```python
from build123d import *

# Parameters (mm, degrees)
BOSS_EXTRUDE2_DEPTH = 5
SKETCH5_R           = 4
BOSS_EXTRUDE3_DEPTH = 7
SKETCH6_R           = 15.5
CUT_EXTRUDE1_DEPTH  = 4
SKETCH7_R           = 1.8
CUT_EXTRUDE2_DEPTH  = 4
CUT_EXTRUDE3_DEPTH  = 6
CUT_EXTRUDE4_DEPTH  = 7
SKETCH11_R          = 4
BOSS_EXTRUDE4_DEPTH = 7
SKETCH12_R          = 42.5
BOSS_EXTRUDE5_DEPTH = 5
SKETCH13_R          = 45.773900861
SKETCH13_R_2        = 42.5
CUT_EXTRUDE5_DEPTH  = 5
SKETCH14_R          = 16
CUT_EXTRUDE6_DEPTH  = 2.5
SKETCH15_R          = 1.7
CUT_EXTRUDE7_DEPTH  = 2.5
CUT_EXTRUDE8_START  = -14
CUT_EXTRUDE8_DEPTH  = 14
FILLET1_R           = 20


with BuildPart() as part:
    # Sketch4 → Boss-Extrude2 (new body)
    with BuildSketch(Plane.XY):
        with BuildLine():
            Line((-17, 0), (-17, 34))
            Line((-17, 34), (17, 34))
            Line((17, 34), (17, 0))
            ThreePointArc((17, 0), (0, -17), (-17, 0))
        make_face()
    extrude(amount=BOSS_EXTRUDE2_DEPTH)

    # Sketch5 → Boss-Extrude3 (add)
    with BuildSketch(Plane.XY.offset(5)):
        with Locations(Location((0, -8.5, 0), (0, 0, 180))):
            Circle(SKETCH5_R)
    extrude(amount=BOSS_EXTRUDE3_DEPTH)

    # Sketch6 → Cut-Extrude1 (cut)
    with BuildSketch(Plane(origin=(0, 0, 0), x_dir=(-1, 0, 0), z_dir=(0, 0, -1))):
        with Locations((0, 17.71586122)):
            Circle(SKETCH6_R)
    extrude(amount=-CUT_EXTRUDE1_DEPTH, mode=Mode.SUBTRACT)

    # Sketch7 → Cut-Extrude2 (cut)
    with BuildSketch(Plane(origin=(0, 0, 4), x_dir=(-1, 0, 0), z_dir=(0, 0, -1))):
        with Locations((0, 17.71586122)):
            Circle(SKETCH7_R)
    extrude(amount=-CUT_EXTRUDE2_DEPTH, mode=Mode.SUBTRACT)

    # Sketch8 → Cut-Extrude3 (cut)
    with BuildSketch(Plane.XY.offset(12)):
        with BuildLine():
            Line((-1.405880507, -7.12), (1.405880507, -7.12))
            ThreePointArc((1.405880507, -7.12), (0, -10.47), (-1.405880507, -7.12))
        make_face()
    extrude(amount=-CUT_EXTRUDE3_DEPTH, mode=Mode.SUBTRACT)

    # Sketch10 → Cut-Extrude4 (cut)
    with BuildSketch(Plane.XY.offset(12)):
        with BuildLine():
            Line((1.439062195, -7.04), (-1.439062195, -7.04))
            ThreePointArc((-1.439062195, -7.04), (0, -10.55), (1.439062195, -7.04))
        make_face()
    extrude(amount=-CUT_EXTRUDE4_DEPTH, mode=Mode.SUBTRACT)

    # Sketch11 → Boss-Extrude4 (add)
    with BuildSketch(Plane.XY.offset(12)):
        with Locations(Location((0, -8.5, 0), (0, 0, 180))):
            Circle(SKETCH11_R)
        with BuildLine():
            Line((1.439062195, -7.04), (-1.439062195, -7.04))
            ThreePointArc((-1.439062195, -7.04), (0, -10.55), (1.439062195, -7.04))
        make_face(mode=Mode.SUBTRACT)
    extrude(amount=BOSS_EXTRUDE4_DEPTH)

    # Sketch12 → Boss-Extrude5 (add)
    with BuildSketch(Plane.XY.offset(5)):
        with Locations((0, -8.5)):
            Circle(SKETCH12_R)
    extrude(amount=-BOSS_EXTRUDE5_DEPTH)

    # Sketch13 → Cut-Extrude5 (cut)
    with BuildSketch(Plane.XY.offset(5)):
        with Locations((0, -8.5)):
            Circle(SKETCH13_R)
        with Locations((0, -8.5)):
            Circle(SKETCH13_R_2, mode=Mode.SUBTRACT)
    extrude(amount=-CUT_EXTRUDE5_DEPTH, mode=Mode.SUBTRACT)

    # Sketch14 → Cut-Extrude6 (cut)
    with BuildSketch(Plane(origin=(0, 0, 0), x_dir=(-1, 0, 0), z_dir=(0, 0, -1))):
        with Locations((0, 16)):
            Circle(SKETCH14_R)
        with Locations(Location((0, -33, 0), (0, 0, 180))):
            Circle(SKETCH14_R)
        with Locations((-24.5, -8.5)):
            Circle(SKETCH14_R)
        with Locations(Location((24.5, -8.5, 0), (0, 0, 180))):
            Circle(SKETCH14_R)
    extrude(amount=-CUT_EXTRUDE6_DEPTH, mode=Mode.SUBTRACT)

    # Sketch15 → Cut-Extrude7 (cut)
    with BuildSketch(Plane(origin=(0, 0, 2.5), x_dir=(-1, 0, 0), z_dir=(0, 0, -1))):
        with Locations((0, 16)):
            Circle(SKETCH15_R)
        with Locations((-24.5, -8.5)):
            Circle(SKETCH15_R)
        with Locations((24.5, -8.5)):
            Circle(SKETCH15_R)
        with Locations((0, -33)):
            Circle(SKETCH15_R)
    extrude(amount=-CUT_EXTRUDE7_DEPTH, mode=Mode.SUBTRACT)

    # Sketch16 → Cut-Extrude8 (cut)
    with BuildSketch(Plane.XY.offset(19).offset(CUT_EXTRUDE8_START)):
        with BuildLine():
            Line((1.803025236, -6.04), (-1.803025236, -6.04))
            ThreePointArc((-1.803025236, -6.04), (0, -11.55), (1.803025236, -6.04))
        make_face()
        with BuildLine():
            Line((1.439062195, -7.04), (-1.439062195, -7.04))
            ThreePointArc((-1.439062195, -7.04), (0, -10.55), (1.439062195, -7.04))
        make_face(mode=Mode.SUBTRACT)
    extrude(amount=CUT_EXTRUDE8_DEPTH, mode=Mode.SUBTRACT)

    # Fillet1
    # the kernel refuses this fillet: 20 mm, written as the material it adds along each edge
    with BuildSketch(Plane(origin=(0, -8.5, 5), x_dir=(-1, 0, 0), z_dir=(0, 1, 0))) as fillet1_piece_1_section:
        with BuildLine():
            CenterArc((23.078784028, 20), FILLET1_R, 197.457603124, 72.542396876)
            Line((4, 14), (3.618424319, 13.88))
            ThreePointArc((3.618424319, 13.88), (3.6, 7), (3.6, 0))
            Line((3.6, 0), (4, -0.4))
            Line((4, -0.4), (23.078784028, -0.4))
            Line((23.078784028, -0.4), (23.078784028, 0))
        make_face()
    fillet1_piece_1 = revolve(axis=Axis((0, -8.5, 5), (0, 0, 1)), mode=Mode.PRIVATE)
    fillet1_piece_1 = fillet1_piece_1 - Plane(origin=(0, -33, 8.742108551), x_dir=(-1, 0, 0), z_dir=(0, 0, -1)) * Cylinder(1.7, 93, mode=Mode.PRIVATE)
    fillet1_piece_1 = fillet1_piece_1 - Plane(origin=(-24.5, -8.5, 8.742108551), x_dir=(-1, 0, 0), z_dir=(0, 0, -1)) * Cylinder(1.7, 93, mode=Mode.PRIVATE)
    fillet1_piece_1 = fillet1_piece_1 - Plane(origin=(0, 16, 8.742108551), x_dir=(-1, 0, 0), z_dir=(0, 0, -1)) * Cylinder(1.7, 93, mode=Mode.PRIVATE)
    fillet1_piece_1 = fillet1_piece_1 - Plane(origin=(24.5, -8.5, 8.742108551), x_dir=(-1, 0, 0), z_dir=(0, 0, -1)) * Cylinder(1.7, 93, mode=Mode.PRIVATE)
    add(fillet1_piece_1)


solid = part.part
```
Geometry: final body of the model. Coordinates: model frame, mm. A direction names the side the tool comes from. Give positions to 0.01 mm unless a question says otherwise; leave off trailing zeros. Write each loop counter-clockwise with the first axis right and the second up, starting at its lowest first coordinate (ties: lowest second). Pieces come first, ordered by that corner, then holes.
1. Section query B-B, the plane x = 25. Return loops of the section in (y, z), then the cut area to 3 significant figures.
2. Pin query (flat end, axial travel): P1, Ø8, axis at y = -39, z = 2.5, coming from the -X side; P2, Ø1.1, axis at x = 0.5, z = 13, coming from the -Y side; P3, Ø9.5, axis at x = 21.5, y = -7, coming from the -Z side. Return the tip coordinate at first contact, or that it passes through.
3. Section query A-A, the plane y = -33. Return loops of the section in (x, z).
4. Draft query along X for faces 1 (the cylindrical face through (30.622, 20.971, 2.535)), 2 (the cylindrical face through (3.47, 0.38, 1.23)), 3 (the flat face through (0.06, -5.89, 19)). Return one class per face: released by +X, released by -X, zero draft, split by the parting line, or undercut.
5. Section query C-C, the plane z = 1. Return loops of the section in (x, y), then the cut area to 3 significant figures.
6. Section query D-D, the plane z = 7.75. Return loops of the section in (x, y), then the cut area to 3 significant figures.
7. Reachability of faces 4 (the flat face through (0, -6.04, 12)), 5 (the cylindrical face through (-27.97, 7.12, 1.23)), 6 (the cylindrical face through (22.89, -7.95, 3.73)) from +Z, -Z, +X, -X, +Y, -Y: full face, straight path, thin tool, end or side. Return the list, or none.
8. Line query: probe 1 along Y at (x, z) = (0, 3.4); probe 2 along Y at (x, z) = (0, 1.35); probe 3 along Z at (x, y) = (-19, 16.5). Output: solid intervals per line, ascending.
Computed:
1. outline: (-42.87, 0) - (-24.49, 0) - (-24.49, 2.5) - (-10.12, 2.5) - (-10.12, 5) - (-42.87, 5) - close; (-6.88, 2.5) - (7.49, 2.5) - (7.49, 0) - (25.87, 0) - (25.87, 5) - (-6.88, 5) - close
1. area: 256 mm2
2. P1: stops at x = -33.23
2. P2: stops at y = -15.99
2. P3: stops at z = 2.5
3. outline: (-34.73, 0) - (-16, 0) - (-16, 2.5) - (-1.7, 2.5) - (-1.7, 5) - (-34.73, 5) - close; (1.7, 2.5) - (16, 2.5) - (16, 0) - (34.73, 0) - (34.73, 5) - (1.7, 5) - close
4. face 1: split by the parting line
4. face 2: undercut
4. face 3: zero draft
5. outline: circle Ø85 at (0, -8.5); hole circle Ø32 at (-24.5, -8.5); hole circle Ø32 at (0, -33); hole circle Ø32 at (0, 16); hole circle Ø32 at (24.5, -8.5)
5. area: 2,460 mm2
6. outline: circle Ø25.92 at (0, -8.5); hole (-1.8, -6.04) arc R3.05 ccw (long way) to (1.8, -6.04) - close
6. area: 500 mm2
7. face 4: +Z
7. face 5: -Z
7. face 6: +Z, -Z
8. probe 1: y = -51 to -34.7, -31.3 to 14.3, 17.7 to 34
8. probe 2: y = -51 to -49, -17 to 0, 32 to 34
8. probe 3: z = 0 to 5
